Can you work these out from the model? Positions are in its coordinate system, mm. Give positions to 0.01 mm unless a question says otherwise; leave off trailing zeros. Write each loop counter-clockwise with the first axis right and the second up, starting at its lowest first coordinate (ties: lowest second). Pieces come first, ordered by that corner, then holes.
Autodesk Fusion 360 part; units mm, degrees
sketch "Sketch1" plane through (0, 0, 0) normal (0, 0, 1) x (1, 0, 0)
  line L0 (-35, 10) -> (35, 10)
  line L1 (35, 10) -> (35, -10)
  line L2 (35, -10) -> (-15, -60)
  line L3 (-15, -60) -> (-35, -60)
  line L4 (-35, -60) -> (-35, 10)
  point P0 (35, 0)
  point P1 (0, 10)
  dimension "d2" = 50
  dimension "d3" = 20
  dimension "d4" = 45
  dimension "d5" = 20
extrude "Extrude1" add sketch "Sketch1" along normal blind 5
sketch "Sketch2" plane through (0, 0, 5) normal (0, 0, 1) x (-1, 0, 0)
  line L0 (35, 60) -> (15, 60)
  line L1 (15, 60) -> (-35, 10)
  line L2 (-35, 10) -> (-35, -10)
  line L3 (-35, -10) -> (35, -10)
  line L4 (35, -10) -> (35, 60)
  circle A0 centre (-20, 0) radius 2.7
  circle A1 centre (20, 0) radius 2.7
  dimension "d8" = 5.4
  dimension "d9" = 5.4
  dimension "d10" = 20
  dimension "d11" = 20
extrude "Extrude2" cut sketch "Sketch2" against normal blind 10 contours A0 | A1
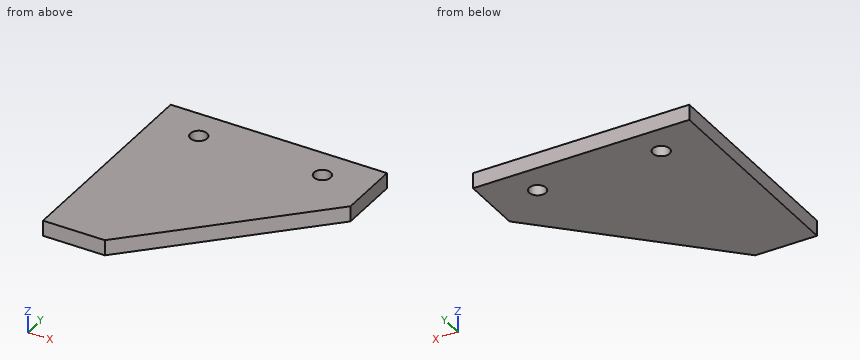
1) Please list where these lines run through material, in increasing order: L1, parallel to X at y = 0, z = 2.55; L2, parallel to Y at x = -20, z = 2.25; L3, parallel to Y at x = 20, z = 2.4.
Values follow:
L1: x = -35 to -22.7, -17.3 to 17.3, 22.7 to 35
L2: y = -60 to -2.7, 2.7 to 10
L3: y = -25 to -2.7, 2.7 to 10
2) For pin 1 Ø8.5 at (x, y) = (20, 0) entering from +Z; pin 2 Ø5 at (x, y) = (-20, 0) entering from +Z, each with a flat end and sliding along its axis, tell me the tip position at first contact or that it passes through.
Values follow:
pin 1: stops at z = 5
pin 2: passes through
3) Suppose I cut it at D-D on x = 20. Write out the boundary of the cut face in (y, z), plus the area to 3 significant figures.
Values follow:
outline: (-25, 0) - (-2.7, 0) - (-2.7, 5) - (-25, 5) - close; (2.7, 0) - (10, 0) - (10, 5) - (2.7, 5) - close
area: 148 mm2
4) Suppose I cut it at A-A on x = -20. Write out the boundary of the cut face in (y, z).
Values follow:
outline: (-60, 0) - (-2.7, 0) - (-2.7, 5) - (-60, 5) - close; (2.7, 0) - (10, 0) - (10, 5) - (2.7, 5) - close
5) Suppose I cut it at B-B on y = 0. Write out the boundary of the cut face in (x, z), plus the area to 3 significant figures.
Values follow:
outline: (-35, 0) - (-22.7, 0) - (-22.7, 5) - (-35, 5) - close; (-17.3, 0) - (17.3, 0) - (17.3, 5) - (-17.3, 5) - close; (22.7, 0) - (35, 0) - (35, 5) - (22.7, 5) - close
area: 296 mm2
6) Suppose I cut it at C-C on z = 2.25. Write out the boundary of the cut face in (x, y).
Values follow:
outline: (-35, -60) - (-15, -60) - (35, -10) - (35, 10) - (-35, 10) - close; hole circle Ø5.4 at (-20, 0); hole circle Ø5.4 at (20, 0)
